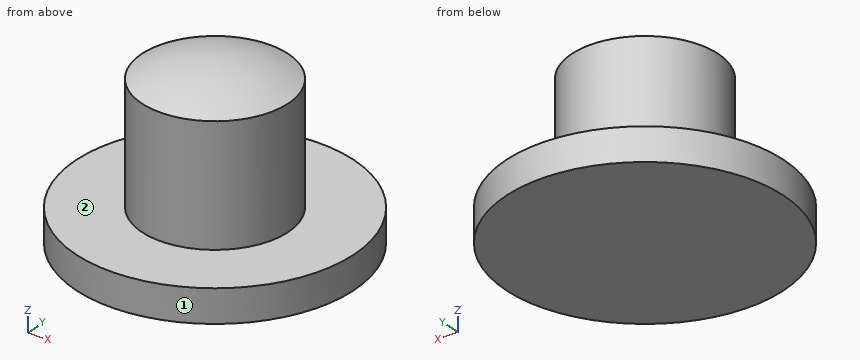
```python
from build123d import *

# Parameters (mm, degrees)
CYLINDER001_R     = 19
CYLINDER001_DEPTH = 4.5
CYLINDER_R        = 10
CYLINDER_DEPTH    = 27


with BuildPart() as cilindro001:
    # Cylinder001 → Cylinder001 (new body)
    with BuildSketch(Plane.XY):
        Circle(CYLINDER001_R)
    extrude(amount=CYLINDER001_DEPTH)


with BuildPart() as cilindro:
    # Cylinder → Cylinder (new body)
    with BuildSketch(Plane.XY):
        Circle(CYLINDER_R)
    extrude(amount=CYLINDER_DEPTH)


with BuildPart() as fusion:
    # Sphere → Sphere (revolve)
    with BuildSketch(Plane.XZ):
        with BuildLine():
            ThreePointArc((23, 0), (16.263456, 16.263456), (0, 23))
            Line((0, 23), (0, 0))
            Line((0, 0), (23, 0))
        make_face()
    revolve(axis=Axis((0, 0, 0), (0, 0, 1)))

    # Common: intersect Cilindro
    add(cilindro.part, mode=Mode.INTERSECT)

    # Fusion: union Cilindro001
    add(cilindro001.part)


solid = fusion.part
```
CAD build for the part. Positions are in the model's coordinates, mm. Face numbers are marked on the shaded views. A direction names the side the tool comes from. Round coordinates to 2 decimals unless told otherwise and drop trailing zeros. Order: outer loops, then holes, each group sorted by start corner. A loop starts at its lowest first (then second) coordinate and runs counter-clockwise, first axis right, second up. Notation, with made-up numbers: (0, -21.75) - (28, -21.75) arc R35 ccw to (28, 14.25) - close; hole circle Ø9 at (-38, 40.25). An arc over 180 degrees is marked (long way). Answer as CSV lines item,"result". Start each with the question number.
1. Saw through at A-A, the plane z = 4. Write the cut outline in (x, y), and give its area (3 significant figures).
2. Tool access for the marked faces 1 and 2: list every direction of +Z, -Z, +X, -X, +Y, -Y with a clear straight run to the whole face (end or side of a thin tool).
3. Saw through at C-C, the plane y = -13. Write the cut outline in (x, z).
4. Drill centre lines: L1, parallel to Z at x = 17.5, y = 2.5; L2, parallel to X at y = 0, z = 5; L3, parallel to Y at x = 1, z = 9.75. Where is each one in solid material? Low to high. Write a range as [from, to].
5. Saw through at B-B, the plane x = -16. Write the cut outline in (y, z).
6. Saw through at D-D, the plane z = 11.5. Write the cut outline in (x, y), and give its area (3 significant figures).
7. Pin check, flat tips, straight feed: pin 1 (6 mm diameter, centred on x = 0, z = 15.5, fed in from +Y); pin 2 (4 mm diameter, centred on y = 5.5, z = 11, fed in from +X); pin 3 (3 mm diameter, centred on x = -12, z = 9.5, fed in from +Y); pin 4 (4 mm diameter, centred on x = 0, z = 3.5, fed in from -Y). Stop position of each tip, or through.
Model answer:
1,outline,"circle Ø38 at (0, 0)"
1,area,"1,130 mm²"
2,face 1,"+Z, -Z"
2,face 2,"+Z"
3,outline,"(-13.86, 0) - (13.86, 0) - (13.86, 4.5) - (-13.86, 4.5) - close"
4,L1,"z = [0, 4.5]"
4,L2,"x = [-10, 10]"
4,L3,"y = [-9.95, 9.95]"
5,outline,"(-10.25, 0) - (10.25, 0) - (10.25, 4.5) - (-10.25, 4.5) - close"
6,outline,"circle Ø20 at (0, 0)"
6,area,"314 mm²"
7,pin 1,"stops at y = 10"
7,pin 2,"stops at x = 9.37"
7,pin 3,"passes through"
7,pin 4,"stops at y = -19"
